```python
from build123d import *

# Parameters (mm, degrees)
BOSS_EXTRUDE1_DEPTH = 19.05
CUT_EXTRUDE2_REACH  = 59.15
SKETCH3_R           = 3.3274
CUT_EXTRUDE3_REACH  = 59.15
SKETCH4_R           = 3.3274
CUT_EXTRUDE1_REACH  = 37.381
FILLET1_R           = 1.27


with BuildPart() as part:
    # Sketch1 → Boss-Extrude1 (new, symmetric)
    with BuildSketch(Plane.XY):
        Polygon((0, 0), (0, 38.1), (-4.064, 38.1), (-38.1, 4.064), (-38.1, 0), align=None)
        Polygon((-32.352636083, 4.064), (-4.064, 4.064), (-4.064, 32.352636083), align=None, mode=Mode.SUBTRACT)
    extrude(amount=BOSS_EXTRUDE1_DEPTH, both=True)

    # Sketch3 → Cut-Extrude2 (cut, up to next)
    with BuildSketch(Plane(origin=(0, 0, 0), x_dir=(0, 0, -1), z_dir=(1, 0, 0)), mode=Mode.PRIVATE) as cut_extrude2_sk1:
        with Locations(Location((0, 19.05, 0), (0, 0, 90))):
            Circle(SKETCH3_R)
    cut_extrude2_tool1 = extrude(cut_extrude2_sk1.sketch, amount=-CUT_EXTRUDE2_REACH, mode=Mode.PRIVATE) & part.part
    add(cut_extrude2_tool1.solids().sort_by_distance((0, 19.05, 0))[0], mode=Mode.SUBTRACT)

    # Sketch4 → Cut-Extrude3 (cut, up to next)
    with BuildSketch(Plane.XZ, mode=Mode.PRIVATE) as cut_extrude3_sk1:
        with Locations(Location((-19.05, 0, 0), (0, 0, 270))):
            Circle(SKETCH4_R)
    cut_extrude3_tool1 = extrude(cut_extrude3_sk1.sketch, amount=-CUT_EXTRUDE3_REACH, mode=Mode.PRIVATE) & part.part
    add(cut_extrude3_tool1.solids().sort_by_distance((-19.05, 0, 0))[0], mode=Mode.SUBTRACT)

    # Sketch2 → Cut-Extrude1 (cut, up to next)
    with BuildSketch(Plane(origin=(-21.082, 21.082, 0), x_dir=(0, 0, 1), z_dir=(-0.7071067811865477, 0.7071067811865475, 0)), mode=Mode.PRIVATE) as cut_extrude1_sk1:
        with BuildLine():
            Line((3.81, 16.447086404), (-3.81, 16.447086404))
            ThreePointArc((-3.81, 16.447086404), (-9.198153673, 14.215240077), (-11.43, 8.827086404))
            Line((-11.43, 8.827086404), (-11.43, -8.827086404))
            ThreePointArc((-11.43, -8.827086404), (-9.198153673, -14.215240077), (-3.81, -16.447086404))
            Line((-3.81, -16.447086404), (3.81, -16.447086404))
            ThreePointArc((3.81, -16.447086404), (9.198153673, -14.215240077), (11.43, -8.827086404))
            Line((11.43, -8.827086404), (11.43, 8.827086404))
            ThreePointArc((11.43, 8.827086404), (9.198153673, 14.215240077), (3.81, 16.447086404))
        make_face()
    cut_extrude1_tool1 = extrude(cut_extrude1_sk1.sketch, amount=-CUT_EXTRUDE1_REACH, mode=Mode.PRIVATE) & part.part
    add(cut_extrude1_tool1.solids().sort_by_distance((-21.082, 21.082, 0))[0], mode=Mode.SUBTRACT)

    # Fillet1
    fillet1_edges = [part.edges().sort_by_distance(p)[0] for p in [
        (-4.064, 4.064, 0),
        (-4.064, 32.352636083, 0),
        (-32.352636083, 4.064, 0),
        (-38.1, 0, 0),
        (-38.1, 4.064, 0),
        (-4.064, 38.1, 0),
        (0, 38.1, 0),
        (0, 0, 0),
    ]]
    fillet(fillet1_edges, radius=FILLET1_R)


solid = part.part
```
Geometry: final body of the model. Coordinates: model frame, mm. A direction names the side the tool comes from. Round coordinates to 2 decimals unless told otherwise and drop trailing zeros. Write each loop counter-clockwise with the first axis right and the second up, starting at its lowest first coordinate (ties: lowest second). Pieces come first, ordered by that corner, then holes.
Item 1: Material intervals for L1, parallel to X at y = 2.05, z = 0; L2, parallel to Z at x = -2, y = 19; L3, parallel to Y at x = -21.5, z = 10.5, sorted ascending.
Item 2: Section query C-C (x = -19.05). Return loops of the section in (y, z), plus the area to 3 significant figures.
Item 3: Set-up query: faces 4 (the face through (-9.572, 29.759, -9.139)), 5 (the face through (-29.759, 9.572, 9.139)), 6 (the face through (-30.452, 4.829, 0.267)). Return all of +Z, -Z, +X, -X, +Y, -Y with unobstructed straight access to the full face (end or side cutting, diameter ignored); none if empty.
Item 4: Section query B-B (z = 0). Return loops of the section in (x, y).
Item 5: Section query D-D (x = -2.5). Return loops of the section in (y, z).
Item 6: Mould query, pull axis Z, two halves, no side actions, for faces 1 (the face through (-16, 21, 19.05)), 2 (the face through (-4.446, 4.426, -0.267)), 3 (the face through (-29.675, 9.656, -9.257)). Classes: +Z half, -Z half, draft (parallel to the pull), parting line (faces both ways), or undercut.
Item 7: Pin query (flat end, axial travel): P1, Ø5.5, axis at x = -19.05, z = 0, coming from the -Y side; P2, Ø3, axis at x = -32, z = 11, coming from the +Y side; P3, Ø8, axis at x = -32.5, z = 9.5, coming from the +Y side; P4, Ø6, axis at y = 26.5, z = 7.5, coming from the -X side. Return the tip coordinate at first contact, or that it passes through.
Item 8: Section query A-A (z = 16.5). Return loops of the section in (x, y).
Completed:
1. L1: x = -38.1 to -22.38, -15.72 to 0
1. L2: z = -19.05 to -3.33, 3.33 to 19.05
1. L3: y = 0 to 4.06
2. outline: (0, -19.05) - (4.06, -19.05) - (4.06, -3.33) - (0, -3.33) - close; (0, 3.33) - (4.06, 3.33) - (4.06, 19.05) - (0, 19.05) - close; (17.37, -19.05) - (23.11, -19.05) - (23.11, -11.43) - (17.37, -11.43) - close; (17.37, 11.43) - (23.11, 11.43) - (23.11, 19.05) - (17.37, 19.05) - close
2. area: 215 mm2
3. face 4: -X
3. face 5: +Y
3. face 6: +Z, -Z
4. outline: (-38.1, 1.27) arc R1.27 ccw to (-36.83, 0) - (-22.38, 0) - (-22.38, 4.06) - (-29.29, 4.06) arc R1.27 cw to (-30.18, 6.23) - (-29.84, 6.58) - (-32.71, 9.45) - (-37.73, 4.44) arc R1.27 ccw to (-38.1, 3.54) - close; (-15.72, 0) - (-1.27, 0) arc R1.27 ccw to (0, 1.27) - (0, 15.72) - (-4.06, 15.72) - (-4.06, 5.33) arc R1.27 cw to (-5.33, 4.06) - (-15.72, 4.06) - close; (-9.45, 32.71) - (-6.58, 29.84) - (-6.23, 30.18) arc R1.27 cw to (-4.06, 29.29) - (-4.06, 22.38) - (0, 22.38) - (0, 36.83) arc R1.27 ccw to (-1.27, 38.1) - (-3.54, 38.1) arc R1.27 ccw to (-4.44, 37.73) - close
5. outline: (0, -19.05) - (38.1, -19.05) - (38.1, 19.05) - (0, 19.05) - close; hole circle Ø6.65 at (19.05, 0)
6. face 1: +Z half
6. face 2: draft
6. face 3: undercut
7. P1: passes through
7. P2: stops at y = 11.66
7. P3: stops at y = 13.32
7. P4: stops at x = -9.46
8. outline: (-38.1, 1.27) arc R1.27 ccw to (-36.83, 0) - (-1.27, 0) arc R1.27 ccw to (0, 1.27) - (0, 36.83) arc R1.27 ccw to (-1.27, 38.1) - (-3.54, 38.1) arc R1.27 ccw to (-4.44, 37.73) - (-37.73, 4.44) arc R1.27 ccw to (-38.1, 3.54) - close; hole (-30.18, 6.23) arc R1.27 ccw to (-29.29, 4.06) - (-5.33, 4.06) arc R1.27 ccw to (-4.06, 5.33) - (-4.06, 29.29) arc R1.27 ccw to (-6.23, 30.18) - close
